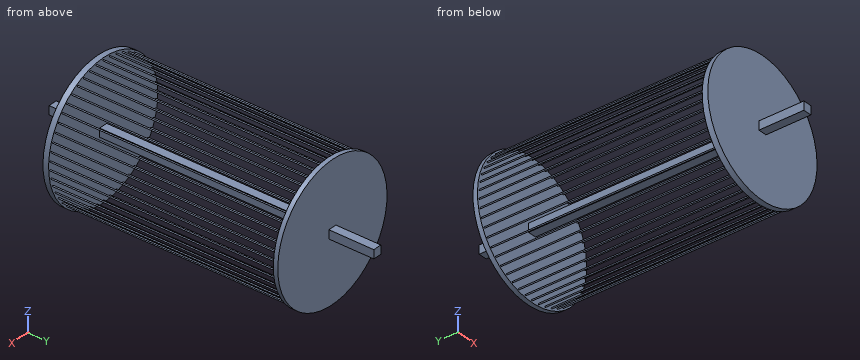
```python
from build123d import *

# Parameters (mm, degrees)
SKETCH1_R           = 76.2
BOSS_EXTRUDE1_DEPTH = 6.35
SKETCH3_W           = 9.7234375
SKETCH3_H           = 9.7234375
BOSS_EXTRUDE2_DEPTH = 254
SKETCH4_R           = 76.2
BOSS_EXTRUDE3_DEPTH = 5.08
SKETCH5_R           = 0.635
BOSS_EXTRUDE4_DEPTH = 254
SKETCH6_W           = 9.7234375
SKETCH6_H           = 9.7234375
BOSS_EXTRUDE5_DEPTH = 50.8
SKETCH7_W           = 9.7234375
SKETCH7_H           = 9.7234375
BOSS_EXTRUDE6_DEPTH = 50.8


with BuildPart() as part:
    # Sketch1 → Boss-Extrude1 (new body)
    with BuildSketch(Plane(origin=(0, 0, 0), x_dir=(1, 0, 0), z_dir=(0, 1, 0))):
        with Locations(Location((0, 0, 0), (0, 0, 270))):
            Circle(SKETCH1_R)
    extrude(amount=BOSS_EXTRUDE1_DEPTH)

    # Sketch3 → Boss-Extrude2 (add)
    with BuildSketch(Plane(origin=(0, 6.35, 0), x_dir=(1, 0, 0), z_dir=(0, 1, 0))):
        Rectangle(SKETCH3_W, SKETCH3_H)
    extrude(amount=BOSS_EXTRUDE2_DEPTH)

    # Sketch4 → Boss-Extrude3 (add)
    with BuildSketch(Plane(origin=(0, 260.35, 0), x_dir=(1, 0, 0), z_dir=(0, 1, 0))):
        with Locations(Location((0, 0, 0), (0, 0, 270))):
            Circle(SKETCH4_R)
    extrude(amount=BOSS_EXTRUDE3_DEPTH)

    # Sketch5 → Boss-Extrude4 (add)
    with BuildSketch(Plane(origin=(0, 6.35, 0), x_dir=(1, 0, 0), z_dir=(0, 1, 0))):
        with Locations(Location((0, 73.66, 0), (0, 0, 270))):
            Circle(SKETCH5_R)
        with Locations(Location((9.232045984, 73.079168899, 0), (0, 0, 270))):
            Circle(SKETCH5_R)
        with Locations(Location((18.318497089, 71.345835649, 0), (0, 0, 270))):
            Circle(SKETCH5_R)
        with Locations(Location((27.116054551, 68.487335951, 0), (0, 0, 270))):
            Circle(SKETCH5_R)
        with Locations(Location((35.485975634, 64.548750052, 0), (0, 0, 270))):
            Circle(SKETCH5_R)
        with Locations(Location((43.296261684, 59.592191806, 0), (0, 0, 270))):
            Circle(SKETCH5_R)
        with Locations(Location((50.423739823, 53.695829096, 0), (0, 0, 270))):
            Circle(SKETCH5_R)
        with Locations(Location((56.756005463, 46.952651085, 0), (0, 0, 270))):
            Circle(SKETCH5_R)
        with Locations(Location((62.193194993, 39.469001718, 0), (0, 0, 270))):
            Circle(SKETCH5_R)
        with Locations(Location((66.649560685, 31.362902617, 0), (0, 0, 270))):
            Circle(SKETCH5_R)
        with Locations(Location((70.05482299, 22.762191806, 0), (0, 0, 270))):
            Circle(SKETCH5_R)
        with Locations(Location((72.355278889, 13.802507632, 0), (0, 0, 270))):
            Circle(SKETCH5_R)
        with Locations(Location((73.514648816, 4.625149669, 0), (0, 0, 270))):
            Circle(SKETCH5_R)
        with Locations(Location((73.514648816, -4.625149668, 0), (0, 0, 270))):
            Circle(SKETCH5_R)
        with Locations(Location((72.355278889, -13.802507632, 0), (0, 0, 270))):
            Circle(SKETCH5_R)
        with Locations(Location((70.05482299, -22.762191806, 0), (0, 0, 270))):
            Circle(SKETCH5_R)
        with Locations(Location((66.649560685, -31.362902617, 0), (0, 0, 270))):
            Circle(SKETCH5_R)
        with Locations(Location((62.193194993, -39.469001718, 0), (0, 0, 270))):
            Circle(SKETCH5_R)
        with Locations(Location((56.756005463, -46.952651085, 0), (0, 0, 270))):
            Circle(SKETCH5_R)
        with Locations(Location((50.423739823, -53.695829096, 0), (0, 0, 270))):
            Circle(SKETCH5_R)
        with Locations(Location((43.296261684, -59.592191806, 0), (0, 0, 270))):
            Circle(SKETCH5_R)
        with Locations(Location((35.485975635, -64.548750052, 0), (0, 0, 270))):
            Circle(SKETCH5_R)
        with Locations(Location((27.116054551, -68.48733595, 0), (0, 0, 270))):
            Circle(SKETCH5_R)
        with Locations(Location((18.318497089, -71.345835649, 0), (0, 0, 270))):
            Circle(SKETCH5_R)
        with Locations(Location((9.232045985, -73.079168899, 0), (0, 0, 270))):
            Circle(SKETCH5_R)
        with Locations(Location((0, -73.66, 0), (0, 0, 270))):
            Circle(SKETCH5_R)
        with Locations(Location((-9.232045984, -73.079168899, 0), (0, 0, 270))):
            Circle(SKETCH5_R)
        with Locations(Location((-18.318497088, -71.345835649, 0), (0, 0, 270))):
            Circle(SKETCH5_R)
        with Locations(Location((-27.116054551, -68.487335951, 0), (0, 0, 270))):
            Circle(SKETCH5_R)
        with Locations(Location((-35.485975634, -64.548750052, 0), (0, 0, 270))):
            Circle(SKETCH5_R)
        with Locations(Location((-43.296261684, -59.592191806, 0), (0, 0, 270))):
            Circle(SKETCH5_R)
        with Locations(Location((-50.423739823, -53.695829096, 0), (0, 0, 270))):
            Circle(SKETCH5_R)
        with Locations(Location((-56.756005463, -46.952651085, 0), (0, 0, 270))):
            Circle(SKETCH5_R)
        with Locations(Location((-62.193194992, -39.469001718, 0), (0, 0, 270))):
            Circle(SKETCH5_R)
        with Locations(Location((-66.649560684, -31.362902617, 0), (0, 0, 270))):
            Circle(SKETCH5_R)
        with Locations(Location((-70.05482299, -22.762191806, 0), (0, 0, 270))):
            Circle(SKETCH5_R)
        with Locations(Location((-72.355278889, -13.802507632, 0), (0, 0, 270))):
            Circle(SKETCH5_R)
        with Locations(Location((-73.514648816, -4.625149669, 0), (0, 0, 270))):
            Circle(SKETCH5_R)
        with Locations(Location((-73.514648816, 4.625149668, 0), (0, 0, 270))):
            Circle(SKETCH5_R)
        with Locations(Location((-72.355278889, 13.802507632, 0), (0, 0, 270))):
            Circle(SKETCH5_R)
        with Locations(Location((-70.05482299, 22.762191806, 0), (0, 0, 270))):
            Circle(SKETCH5_R)
        with Locations(Location((-66.649560685, 31.362902617, 0), (0, 0, 270))):
            Circle(SKETCH5_R)
        with Locations(Location((-62.193194992, 39.469001718, 0), (0, 0, 270))):
            Circle(SKETCH5_R)
        with Locations(Location((-56.756005463, 46.952651085, 0), (0, 0, 270))):
            Circle(SKETCH5_R)
        with Locations(Location((-50.423739823, 53.695829096, 0), (0, 0, 270))):
            Circle(SKETCH5_R)
        with Locations(Location((-43.296261684, 59.592191806, 0), (0, 0, 270))):
            Circle(SKETCH5_R)
        with Locations(Location((-35.485975634, 64.548750052, 0), (0, 0, 270))):
            Circle(SKETCH5_R)
        with Locations(Location((-27.116054551, 68.48733595, 0), (0, 0, 270))):
            Circle(SKETCH5_R)
        with Locations(Location((-18.318497089, 71.345835649, 0), (0, 0, 270))):
            Circle(SKETCH5_R)
        with Locations(Location((-9.232045984, 73.079168899, 0), (0, 0, 270))):
            Circle(SKETCH5_R)
    extrude(amount=BOSS_EXTRUDE4_DEPTH)

    # Sketch6 → Boss-Extrude5 (add)
    with BuildSketch(Plane(origin=(0, 265.43, 0), x_dir=(1, 0, 0), z_dir=(0, 1, 0))):
        Rectangle(SKETCH6_W, SKETCH6_H)
    extrude(amount=BOSS_EXTRUDE5_DEPTH)

    # Sketch7 → Boss-Extrude6 (add)
    with BuildSketch(Plane.XZ):
        Rectangle(SKETCH7_W, SKETCH7_H)
    extrude(amount=BOSS_EXTRUDE6_DEPTH)


solid = part.part
```
Source: CAD feature listing. Evaluate the final solid. Frame: model axes, mm. Coordinates: 2 decimals unless noted, no trailing zeros. Loops run counter-clockwise (first coordinate to the right, second up) from the corner with the lowest first, then second, coordinate; pieces in that order, holes last. Notation, with made-up numbers: M 0,41.5 L 56,41.5 A20 ccw 56,46.5 Z; hole C -2,26.5 d11. An arc over 180 degrees is marked long. Use a Markdown table: item, result. Add a question column.
Q1. Section query B-B, the plane z = 0. Return loops of the section in (x, y).
Q2. Section query A-A, the plane x = -14. Return loops of the section in (y, z), and give its area (3 significant figures).
Q3. Section query C-C, the plane y = 133.5. State how many separate pieces and enclosed holes the cut face has, and give its area (3 significant figures).
Q4. Material intervals for L1, parallel to Y at x = 63, z = 15.5; L2, parallel to Z at x = -35.5, y = 169; L3, parallel to X at y = 11, z = -3, sorted ascending.
Q5. First-contact query: pin 1 (10.5 mm diameter, centred on y = 141, z = 1, fed in from -X); pin 2 (1 mm diameter, centred on y = 231, z = -32, fed in from +X); pin 3 (8 mm diameter, centred on y = 294, z = 0, fed in from -X); pin 4 (2 mm diameter, centred on x = 60.5, y = 117, fed in from -Z). Flat tips, straight axial feed; report the tip coordinate or a pass-through.
Result:
| question | item | result |
|---|---|---|
| 1 | outline | M -76.2,0 L -4.86,0 L -4.86,-50.8 L 4.86,-50.8 L 4.86,0 L 76.2,0 L 76.2,6.35 L 4.86,6.35 L 4.86,260.35 L 76.2,260.35 L 76.2,265.43 L 4.86,265.43 L 4.86,316.23 L -4.86,316.23 L -4.86,265.43 L -76.2,265.43 L -76.2,260.35 L -4.86,260.35 L -4.86,6.35 L -76.2,6.35 Z |
| 2 | outline | M 0,-74.9 L 6.35,-74.9 L 6.35,74.9 L 0,74.9 Z; M 260.35,-74.9 L 265.43,-74.9 L 265.43,74.9 L 260.35,74.9 Z |
| 2 | area | 1,710 mm2 |
| 3 | separate pieces | 51 |
| 3 | enclosed holes | 0 |
| 3 | area | 158 mm2 |
| 4 | L1 | y = 0 to 6.35, 260.35 to 265.43 |
| 4 | L2 | z = -65.18 to -63.91, 63.91 to 65.18 |
| 4 | L3 | x = -4.86 to 4.86 |
| 5 | pin 1 | stops at x = -74.15 |
| 5 | pin 2 | stops at x = 67.27 |
| 5 | pin 3 | stops at x = -4.86 |
| 5 | pin 4 | passes through |
